The listing builds one solid part. Answer for the finished solid, in the listing's coordinates (mm). A direction names the side the tool comes from. Coordinates: 2 decimals unless noted, no trailing zeros. Write each loop counter-clockwise with the first axis right and the second up, starting at its lowest first coordinate (ties: lowest second). Pieces come first, ordered by that corner, then holes.
(1) Which of the six approach directions +Z, -Z, +X, -X, +Y, -Y give full straight-line access (tool end or side, diameter ignored) to faces 1 (the flat face through (32.58, 8.21, 8.96)), 2 (the flat face through (29.7, 0.43, 8.96)), 3 (the flat face through (32.96, 0.5, 101.04)), 4 (the flat face through (29, 8, 14.403)), 5 (the flat face through (29, 8, 3.666))?
(2) The part is cut by section A-A on z = 101. Determine the outline of the cut face in (x, y).
(3) Given P1, Ø12, axis at x = 29, z = 76.5, coming from the -Y side; P2, Ø6, axis at x = 20.5, y = 7.5, coming from the -Z side; P3, Ø6, axis at x = 27.5, y = 7, coming from the -Z side; P4, Ø6, axis at x = 25, z = 27.5, coming from the -Y side, each flat-ended and moving along its own axis, determine where each tip first touches the part or whether it passes through.
(4) The part is cut by section C-C on x = 21. Determine the outline of the cut face in (y, z), plus the area to 3 significant figures.
(5) Straight lines are drawn through the part: line 1 (Y direction, x = 30, z = 96.5); line 2 (Y direction, x = 18, z = 29); line 3 (Y direction, x = 18.5, z = 77.5). For each, find the intervals that lie inside material, in ascending order.
(6) The part is cut by section D-D on y = 21.75. Determine the outline of the cut face in (x, z).
(7) For a pull along X with two mould halves and no side action, classify faces 6 (the flat face through (4.791, 5.766, 54.23)), 7 (the cylindrical face through (33.05, 5.33, 100.89)), 8 (the flat face through (32.58, 8.21, 100.89)), 9 (the flat face through (29, 8, 106.334)) as +X half, -X half, draft (parallel to the pull), parting line (faces both ways), or undercut.
(8) The part is cut by section B-B on y = 5.5. Determine the outline of the cut face in (x, z), plus the area to 3 significant figures.
from build123d import *

# Parameters (mm, degrees)
BOSS_EXTRUDE1_DEPTH = 110
SKETCH3_W           = 6
SKETCH3_H           = 10.73706506
BOSS_EXTRUDE3_DEPTH = 14
SKETCH18_R          = 2.8
CUT_EXTRUDE4_DEPTH  = 117.507131621


with BuildPart() as part:
    # Sketch1 → Boss-Extrude1 (new body)
    with BuildSketch(Plane.XY):
        Polygon((0, 0), (9.717159864, 11.695735532), (18.078758039, 15.773959455), (37.597840156, 25.294051902), (40.338683398, 19.674490473), align=None)
    extrude(amount=BOSS_EXTRUDE1_DEPTH)

    # Sketch3 → Boss-Extrude3 (add)
    with BuildSketch(Plane(origin=(0, 0, 0), x_dir=(0.8987940462991665, 0.43837114678907857, 0), z_dir=(0.43837114678907857, -0.8987940462991665, 0))):
        with Locations((29.880897425, 100.965437953)):
            Rectangle(SKETCH3_W, SKETCH3_H)
        with Locations((29.880897425, 9.034562047)):
            Rectangle(SKETCH3_W, SKETCH3_H)
    extrude(amount=BOSS_EXTRUDE3_DEPTH)

    # Sketch18 → Cut-Extrude4 (cut, through all)
    with BuildSketch(Plane(origin=(0, 0, 3.666029517), x_dir=(-1, 0, 0), z_dir=(0, 0, -1))):
        with Locations((-30.580685329, 4.011697799)):
            Circle(SKETCH18_R)
    extrude(amount=-CUT_EXTRUDE4_DEPTH, mode=Mode.SUBTRACT)


solid = part.part
Model answer:
1. face 1: +Z, -Z, +X
1. face 2: +Z, -Z, -Y
1. face 3: +Z, -Z, +X, -Y
1. face 4: +X, -Y
1. face 5: -Z, +X, -Y
2. outline: (0, 0) - (24.16, 11.78) - (27.8, 4.33) arc R2.8 cw (long way) to (29.11, 1.63) - (30.3, -0.8) - (35.69, 1.83) - (29.55, 14.41) - (40.34, 19.67) - (37.6, 25.29) - (9.72, 11.7) - close
3. P1: stops at y = 11.22
3. P2: stops at z = 0
3. P3: stops at z = 3.67
3. P4: stops at y = 10.73
4. outline: (10.24, 0) - (17.2, 0) - (17.2, 110) - (10.24, 110) - close
4. area: 765 mm2
5. line 1: y = -0.19 to 1.27, 6.75 to 13.5, 14.63 to 21.59
5. line 2: y = 8.78 to 15.74
5. line 3: y = 9.02 to 15.98
6. outline: (30.33, 0) - (39.33, 0) - (39.33, 110) - (30.33, 110) - close
7. face 6: -X half
7. face 7: undercut
7. face 8: +X half
7. face 9: draft
8. outline: (4.57, 0) - (11.28, 0) - (11.28, 110) - (4.57, 110) - close; (27.23, 3.67) - (28.21, 3.67) - (28.21, 14.4) - (27.23, 14.4) - close; (27.23, 95.6) - (28.21, 95.6) - (28.21, 106.33) - (27.23, 106.33) - close; (32.95, 3.67) - (33.9, 3.67) - (33.9, 14.4) - (32.95, 14.4) - close; (32.95, 95.6) - (33.9, 95.6) - (33.9, 106.33) - (32.95, 106.33) - close
8. area: 779 mm2
